```python
from build123d import *

# Parameters (mm, degrees)
F1_DEPTH = 25
F2_DEPTH = 25
F4_DEPTH = 3


with BuildPart() as f1:
    # F0 (on Top) → F1 (new body)
    with BuildSketch(Plane.XY):
        with BuildLine():
            ThreePointArc((0.2530346427, -5.4941763231), (0.9677357809, -4.7104657369), (0.1840251947, -3.9957645986))
            ThreePointArc((0.1840251947, -3.9957645986), (-3.4641016151, 2), (3.5524462473, 1.8385118058))
            ThreePointArc((3.5524462473, 1.8385118058), (4.5632508823, 1.517149098), (4.88461359, 2.527953733))
            ThreePointArc((4.88461359, 2.527953733), (2.9794438001, 4.6230849702), (0.2844262333, 5.4926406871))
            ThreePointArc((0.2844262333, 5.4926406871), (-2.6258785407, 4.8326764727), (-4.7631397208, 2.75))
            ThreePointArc((-4.7631397208, 2.75), (-4.6986032782, -2.8588681736), (0.2530346427, -5.4941763231))
        make_face()
        with BuildLine():
            Line((24.2368602792, 52.9794734195), (-4.7631397208, 2.75))
            ThreePointArc((-4.7631397208, 2.75), (-2.6258785407, 4.8326764727), (0.2844262333, 5.4926406871))
            Line((0.2844262333, 5.4926406871), (24.3854467478, 47.2368327324))
            ThreePointArc((24.3854467478, 47.2368327324), (23.501840136, 50.0872127066), (24.2368602792, 52.9794734195))
        make_face()
        with BuildLine():
            ThreePointArc((29.2844262333, 55.7221141066), (26.3741214593, 55.0621498922), (24.2368602792, 52.9794734195))
            ThreePointArc((24.2368602792, 52.9794734195), (23.501840136, 50.0872127066), (24.3854467478, 47.2368327324))
            ThreePointArc((24.3854467478, 47.2368327324), (26.486012872, 45.3376569144), (29.2530346427, 44.7352970964))
            ThreePointArc((29.2530346427, 44.7352970964), (29.9677357809, 45.5190076826), (29.1840251947, 46.2337088209))
            ThreePointArc((29.1840251947, 46.2337088209), (25.5358983849, 52.2294734195), (32.5524462473, 52.0679852253))
            ThreePointArc((32.5524462473, 52.0679852253), (33.5632508823, 51.7466225175), (33.88461359, 52.7574271525))
            ThreePointArc((33.88461359, 52.7574271525), (31.9794438001, 54.8525583897), (29.2844262333, 55.7221141066))
        make_face()
        with BuildLine():
            Line((28.9481851446, 61.1397274573), (24.2368602792, 52.9794734195))
            ThreePointArc((24.2368602792, 52.9794734195), (26.3741214593, 55.0621498922), (29.2844262333, 55.7221141066))
            Line((29.2844262333, 55.7221141066), (30.6802359522, 58.1397274573))
            ThreePointArc((30.6802359522, 58.1397274573), (31.0462613559, 58.5057528611), (31.5462613559, 58.6397274573))
            Line((31.5462613559, 58.6397274573), (48.2368602792, 58.6397274573))
            ThreePointArc((48.2368602792, 58.6397274573), (48.9439670604, 58.9326206762), (49.2368602792, 59.6397274573))
            Line((49.2368602792, 59.6397274573), (49.2368602792, 61.6397274573))
            Line((49.2368602792, 61.6397274573), (49.2368602792, 65.2549511465))
            Line((49.2368602792, 65.2549511465), (49.2368602792, 69.4975918336))
            Line((49.2368602792, 69.4975918336), (49.2368602792, 82.6397274573))
            ThreePointArc((49.2368602792, 82.6397274573), (49.3129807467, 83.0224108897), (49.529753498, 83.3468342385))
            Line((49.529753498, 83.3468342385), (46.529753498, 86.3468342385))
            ThreePointArc((46.529753498, 86.3468342385), (46.3129807467, 86.0224108897), (46.2368602792, 85.6397274573))
            Line((46.2368602792, 85.6397274573), (46.2368602792, 62.6397274573))
            ThreePointArc((46.2368602792, 62.6397274573), (45.9439670604, 61.9326206762), (45.2368602792, 61.6397274573))
            Line((45.2368602792, 61.6397274573), (29.8142105484, 61.6397274573))
            ThreePointArc((29.8142105484, 61.6397274573), (29.3142105484, 61.5057528611), (28.9481851446, 61.1397274573))
        make_face()
        Polygon((49.2368602792, 69.4975918336), (49.2368602792, 65.2549511465), (67.62163659, 83.6397274573), (63.3789959029, 83.6397274573), align=None)
        with BuildLine():
            ThreePointArc((47.2368602792, 86.6397274573), (46.8541768468, 86.5636069899), (46.529753498, 86.3468342385))
            Line((46.529753498, 86.3468342385), (49.529753498, 83.3468342385))
            ThreePointArc((49.529753498, 83.3468342385), (49.8541768468, 83.5636069899), (50.2368602792, 83.6397274573))
            Line((50.2368602792, 83.6397274573), (63.3789959029, 83.6397274573))
            Line((63.3789959029, 83.6397274573), (67.62163659, 83.6397274573))
            Line((67.62163659, 83.6397274573), (87.2368602792, 83.6397274573))
            ThreePointArc((87.2368602792, 83.6397274573), (87.9439670604, 83.9326206762), (88.2368602792, 84.6397274573))
            Line((88.2368602792, 84.6397274573), (88.2368602792, 85.6397274573))
            ThreePointArc((88.2368602792, 85.6397274573), (87.9439670604, 86.3468342385), (87.2368602792, 86.6397274573))
            Line((87.2368602792, 86.6397274573), (47.2368602792, 86.6397274573))
        make_face()
    extrude(amount=F1_DEPTH)

    # F0 (on Top) → F2 (join)
    with BuildSketch(Plane.XY):
        with BuildLine():
            ThreePointArc((47.2368602792, 86.6397274573), (46.8541768468, 86.5636069899), (46.529753498, 86.3468342385))
            Line((46.529753498, 86.3468342385), (49.529753498, 83.3468342385))
            ThreePointArc((49.529753498, 83.3468342385), (49.8541768468, 83.5636069899), (50.2368602792, 83.6397274573))
            Line((50.2368602792, 83.6397274573), (63.3789959029, 83.6397274573))
            Line((63.3789959029, 83.6397274573), (67.62163659, 83.6397274573))
            Line((67.62163659, 83.6397274573), (87.2368602792, 83.6397274573))
            ThreePointArc((87.2368602792, 83.6397274573), (87.9439670604, 83.9326206762), (88.2368602792, 84.6397274573))
            Line((88.2368602792, 84.6397274573), (88.2368602792, 85.6397274573))
            ThreePointArc((88.2368602792, 85.6397274573), (87.9439670604, 86.3468342385), (87.2368602792, 86.6397274573))
            Line((87.2368602792, 86.6397274573), (47.2368602792, 86.6397274573))
        make_face()
        Polygon((49.2368602792, 69.4975918336), (49.2368602792, 65.2549511465), (67.62163659, 83.6397274573), (63.3789959029, 83.6397274573), align=None)
    extrude(amount=-F2_DEPTH)

    # F3 (on face) → F4 (cut, through all)
    with BuildSketch(Plane(origin=(-8.0090454337, 8.0090454337, 0), x_dir=(0.7071067812, 0.7071067812, 0), z_dir=(0.7071067812, -0.7071067812, 0))):
        Polygon((106.9579362494, -25), (80.9579362494, 0), (80.9579362494, -25), align=None)
    extrude(amount=-F4_DEPTH, mode=Mode.SUBTRACT)


solid = f1.part
```
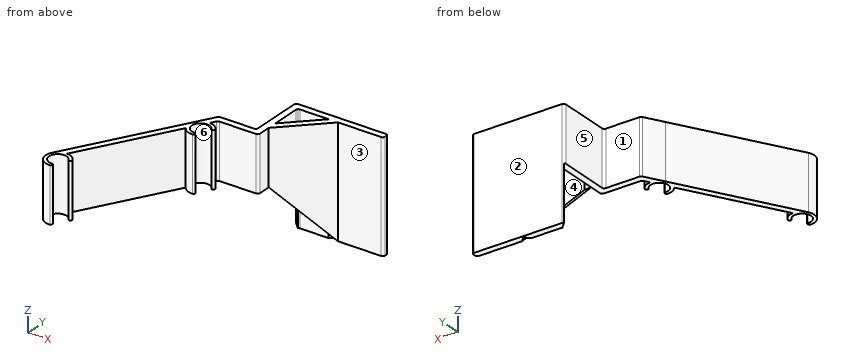
Model file for the job. Use its own axes, mm. Face numbers are marked on the shaded views. A direction names the side the tool comes from. Coordinates: 2 decimals unless noted, no trailing zeros. Loops run counter-clockwise (first coordinate to the right, second up) from the corner with the lowest first, then second, coordinate; pieces in that order, holes last. Notation, with made-up numbers: (-37.5, 16) -> (4.5, 16) arc R6 cw to (4.5, 26) -> close; hole circle Ø3 at (52, 25). An arc over 180 degrees is marked (long way). Answer as a JSON object with one key per item and string values.
Q1. Pull direction X, two halves, no side cores. Call the marked faces 3, 4, 5 and 6: released by +X, released by -X, zero draft, split by the parting line, or undercut.
Report:
{"face 3": "zero draft", "face 4": "undercut", "face 5": "released by -X", "face 6": "undercut"}
Q2. Cut at D-D (x = 35.5). List the corners of the cut face in (y, z), and give its area (3 significant figures).
Report:
{"outline": "(58.64, 0) -> (61.64, 0) -> (61.64, 25) -> (58.64, 25) -> close", "area": "75.0 mm2"}
Q3. Cut at B-B (z = -16.5). List the corners of the cut face in (x, y), and give its area (3 significant figures).
Report:
{"outline": "(46.53, 86.35) -> (49.53, 83.35) arc R1 cw to (50.24, 83.64) -> (63.38, 83.64) -> (59.25, 79.51) -> (61.37, 77.39) -> (67.62, 83.64) -> (87.24, 83.64) arc R1 ccw to (88.24, 84.64) -> (88.24, 85.64) arc R1 ccw to (87.24, 86.64) -> (47.24, 86.64) arc R1 ccw to start", "area": "143 mm2"}
Q4. Cut at C-C (y = 0). List the corners of the cut face in (x, z), and give its area (3 significant figures).
Report:
{"outline": "(-5.5, 0) -> (-4, 0) -> (-4, 25) -> (-5.5, 25) -> close", "area": "37.5 mm2"}
Q5. Probe probe 1 along X at (y, z) = (13.5, 17.5); probe 2 along Y at (x, z) = (0, 20); probe 3 along Y at (x, z) = (69, 5). List the from-to ranges inside material, lowest first.
Report:
{"probe 1": "x = 1.44 to 4.91", "probe 2": "y = -5.5 to -4, 4 to 11", "probe 3": "y = 83.64 to 86.64"}
Q6. 3-axis set-ups, long thin cutter, end or side, ignore diameter. For the marked faces 1 and 2: which of +Z, -Z, +X, -X, +Y, -Y reach the whole face in a straight line?
Report:
{"face 1": "+Z, -Z, -X, +Y", "face 2": "+Z, -Z, +X, -X, +Y"}
Q7. Flat gauge pins, fed straight in: P1, Ø4, axis at y = 71, z = -4.5, coming from the +X side; P2, Ø10.5, axis at x = 57.5, z = 4.5, coming from the -Y side; P3, Ø18.5, axis at y = 77.5, z = 9, coming from the -X side; P4, Ø7, axis at x = 29, y = 50.23, coming from the -Z side. Where does each tip first touch, or does it go through?
Report:
{"P1": "stops at x = 56.98", "P2": "stops at y = 68.27", "P3": "stops at x = 46.24", "P4": "passes through"}
